Can you work these out from the model? Positions are in its coordinate system, mm. Give positions to 0.01 mm unless a question says otherwise; leave off trailing zeros. Write each loop counter-clockwise with the first axis right and the second up, starting at its lowest first coordinate (ties: lowest second). Pieces come first, ordered by that corner, then holes.
1. Suppose I cut it at C-C (x = 6). Please give me the cut outline in (y, z), and give its area (3 significant figures).
2. I'm going to push flat-ended pins straight in: pin 1 (13 mm diameter, centred on x = -29, z = 32, fed in from +Y); pin 2 (2 mm diameter, centred on x = -17, y = 4.5, fed in from -Z). Where does each tip first touch, or does it pass through?
3. Suppose I cut it at A-A (z = 16). Please give me the cut outline in (x, y), and give its area (3 significant figures).
4. If I drill on probe 1 along Z at (x, y) = (-21, 0.95); probe 2 along X at (y, z) = (0.85, 16); probe 3 along Z at (x, y) = (-13, 0.5), over which ranges is the centre line in solid material (lowest first)?
5. Thinking about a two-plate mould opening in Y: for faces 1 (the flat face through (1, 6.16, 0)), 2 (the cylindrical face through (2.479, 1.014, 28.034)), 3 (the cylindrical face through (45, 5, 0)), which applies, pulls with the +Y half, pulls with the -Y half, needs draft (parallel to the pull), parting line crosses it, or undercut?
6. Suppose I cut it at D-D (z = 37.5). Please give me the cut outline in (x, y), and give its area (3 significant figures).
7. Suppose I cut it at B-B (x = -29). Please give me the cut outline in (y, z).
```python
from build123d import *

# Parameters (mm, degrees)
SKETCH1_W               = 100
SKETCH1_H               = 100
BOSS_EXTRUDE1_DEPTH     = 2
BOSS_EXTRUDE2_DEPTH     = 100
FILLET1_R               = 10
SKETCH3_R               = 4
CUT_EXTRUDE1_DEPTH      = 3
LPATTERN1_COUNT         = 5
LPATTERN1_PITCH         = 16
LPATTERN1_COUNT_DIR2    = 2
LPATTERN1_PITCH_DIR2    = 16
MIRROR1_COPY_1_SKETCH_R = 4
MIRROR1_COPY_1_DEPTH    = 3
MIRROR1_COPY_2_SKETCH_R = 4
MIRROR1_COPY_2_DEPTH    = 3
MIRROR1_COPY_3_SKETCH_R = 4
MIRROR1_COPY_3_DEPTH    = 3
MIRROR1_COPY_4_SKETCH_R = 4
MIRROR1_COPY_4_DEPTH    = 3
MIRROR1_COPY_5_SKETCH_R = 4
MIRROR1_COPY_5_DEPTH    = 3
MIRROR1_COPY_6_SKETCH_R = 4
MIRROR1_COPY_6_DEPTH    = 3
MIRROR1_COPY_7_SKETCH_R = 4
MIRROR1_COPY_7_DEPTH    = 3
MIRROR1_COPY_8_SKETCH_R = 4
MIRROR1_COPY_8_DEPTH    = 3
MIRROR1_COPY_9_SKETCH_R = 4
MIRROR1_COPY_9_DEPTH    = 3
SKETCH4_W               = 41.2
SKETCH4_H               = 2
CUT_EXTRUDE2_DEPTH      = 101
SKETCH5_R               = 1
CUT_EXTRUDE3_DEPTH      = 59.8
LPATTERN2_COUNT         = 8
LPATTERN2_PITCH         = 13


with BuildPart() as part:
    # Sketch1 → Boss-Extrude1 (new body)
    with BuildSketch(Plane(origin=(0, 0, 0), x_dir=(1, 0, 0), z_dir=(0, 1, 0))):
        Rectangle(SKETCH1_W, SKETCH1_H)
    extrude(amount=BOSS_EXTRUDE1_DEPTH)

    # Sketch2 → Boss-Extrude2 (add)
    with BuildSketch(Plane(origin=(50, 0, 0), x_dir=(0, 0, -1), z_dir=(1, 0, 0))):
        Polygon((-3.8, 2), (-6.20177712, 6.16), (6.20177712, 6.16), (3.8, 2), align=None)
    extrude(amount=-BOSS_EXTRUDE2_DEPTH)

    # Fillet1
    fillet1_edges = [part.edges().sort_by_distance(p)[0] for p in [
        (50, 1, -50),
        (50, 1, 50),
    ]]
    fillet(fillet1_edges, radius=FILLET1_R)

    # Sketch3 → Cut-Extrude1 (cut, through all)
    with BuildSketch(Plane(origin=(0, 2, 0), x_dir=(1, 0, 0), z_dir=(0, 1, 0))):
        with Locations((35, -16)):
            Circle(SKETCH3_R)
        with Locations((27, -24)):
            Circle(SKETCH3_R)
    cut_extrude1 = extrude(amount=-CUT_EXTRUDE1_DEPTH, mode=Mode.SUBTRACT)

    # LPattern1: Cut-Extrude1 5 × 2
    with Locations(*[(-i * LPATTERN1_PITCH, 0, j * LPATTERN1_PITCH_DIR2) for i in range(LPATTERN1_COUNT) for j in range(LPATTERN1_COUNT_DIR2) if (i, j) != (0, 0)]):
        add(cut_extrude1, mode=Mode.SUBTRACT)

    # Mirror1: Cut-Extrude1 across plane
    add(cut_extrude1.mirror(Plane.XY), mode=Mode.SUBTRACT)

    # Mirror1 copy 1 sketch → Mirror1 copy 1 (cut, through all)
    with BuildSketch(Plane(origin=(0, 2, -16), x_dir=(1, 0, 0), z_dir=(0, 1, 0))):
        with Locations((35, 16)):
            Circle(MIRROR1_COPY_1_SKETCH_R)
        with Locations((27, 24)):
            Circle(MIRROR1_COPY_1_SKETCH_R)
    extrude(amount=-MIRROR1_COPY_1_DEPTH, mode=Mode.SUBTRACT)

    # Mirror1 copy 2 sketch → Mirror1 copy 2 (cut, through all)
    with BuildSketch(Plane(origin=(-16, 2, 0), x_dir=(1, 0, 0), z_dir=(0, 1, 0))):
        with Locations((35, 16)):
            Circle(MIRROR1_COPY_2_SKETCH_R)
        with Locations((27, 24)):
            Circle(MIRROR1_COPY_2_SKETCH_R)
    extrude(amount=-MIRROR1_COPY_2_DEPTH, mode=Mode.SUBTRACT)

    # Mirror1 copy 3 sketch → Mirror1 copy 3 (cut, through all)
    with BuildSketch(Plane(origin=(-16, 2, -16), x_dir=(1, 0, 0), z_dir=(0, 1, 0))):
        with Locations((35, 16)):
            Circle(MIRROR1_COPY_3_SKETCH_R)
        with Locations((27, 24)):
            Circle(MIRROR1_COPY_3_SKETCH_R)
    extrude(amount=-MIRROR1_COPY_3_DEPTH, mode=Mode.SUBTRACT)

    # Mirror1 copy 4 sketch → Mirror1 copy 4 (cut, through all)
    with BuildSketch(Plane(origin=(-32, 2, 0), x_dir=(1, 0, 0), z_dir=(0, 1, 0))):
        with Locations((35, 16)):
            Circle(MIRROR1_COPY_4_SKETCH_R)
        with Locations((27, 24)):
            Circle(MIRROR1_COPY_4_SKETCH_R)
    extrude(amount=-MIRROR1_COPY_4_DEPTH, mode=Mode.SUBTRACT)

    # Mirror1 copy 5 sketch → Mirror1 copy 5 (cut, through all)
    with BuildSketch(Plane(origin=(-32, 2, -16), x_dir=(1, 0, 0), z_dir=(0, 1, 0))):
        with Locations((35, 16)):
            Circle(MIRROR1_COPY_5_SKETCH_R)
        with Locations((27, 24)):
            Circle(MIRROR1_COPY_5_SKETCH_R)
    extrude(amount=-MIRROR1_COPY_5_DEPTH, mode=Mode.SUBTRACT)

    # Mirror1 copy 6 sketch → Mirror1 copy 6 (cut, through all)
    with BuildSketch(Plane(origin=(-48, 2, 0), x_dir=(1, 0, 0), z_dir=(0, 1, 0))):
        with Locations((35, 16)):
            Circle(MIRROR1_COPY_6_SKETCH_R)
        with Locations((27, 24)):
            Circle(MIRROR1_COPY_6_SKETCH_R)
    extrude(amount=-MIRROR1_COPY_6_DEPTH, mode=Mode.SUBTRACT)

    # Mirror1 copy 7 sketch → Mirror1 copy 7 (cut, through all)
    with BuildSketch(Plane(origin=(-48, 2, -16), x_dir=(1, 0, 0), z_dir=(0, 1, 0))):
        with Locations((35, 16)):
            Circle(MIRROR1_COPY_7_SKETCH_R)
        with Locations((27, 24)):
            Circle(MIRROR1_COPY_7_SKETCH_R)
    extrude(amount=-MIRROR1_COPY_7_DEPTH, mode=Mode.SUBTRACT)

    # Mirror1 copy 8 sketch → Mirror1 copy 8 (cut, through all)
    with BuildSketch(Plane(origin=(-64, 2, 0), x_dir=(1, 0, 0), z_dir=(0, 1, 0))):
        with Locations((35, 16)):
            Circle(MIRROR1_COPY_8_SKETCH_R)
        with Locations((27, 24)):
            Circle(MIRROR1_COPY_8_SKETCH_R)
    extrude(amount=-MIRROR1_COPY_8_DEPTH, mode=Mode.SUBTRACT)

    # Mirror1 copy 9 sketch → Mirror1 copy 9 (cut, through all)
    with BuildSketch(Plane(origin=(-64, 2, -16), x_dir=(1, 0, 0), z_dir=(0, 1, 0))):
        with Locations((35, 16)):
            Circle(MIRROR1_COPY_9_SKETCH_R)
        with Locations((27, 24)):
            Circle(MIRROR1_COPY_9_SKETCH_R)
    extrude(amount=-MIRROR1_COPY_9_DEPTH, mode=Mode.SUBTRACT)

    # Sketch4 → Cut-Extrude2 (cut, through all)
    with BuildSketch(Plane.ZY.offset(50)):
        with Locations((-29.4, 1)):
            Rectangle(SKETCH4_W, SKETCH4_H)
    extrude(amount=-CUT_EXTRUDE2_DEPTH, mode=Mode.SUBTRACT)

    # Sketch5 → Cut-Extrude3 (cut, through all)
    with BuildSketch(Plane.XY.offset(50)):
        with Locations((-46, 4)):
            Circle(SKETCH5_R)
    cut_extrude3 = extrude(amount=-CUT_EXTRUDE3_DEPTH, mode=Mode.SUBTRACT)

    # LPattern2: Cut-Extrude3 ×8
    with Locations(*[(i * LPATTERN2_PITCH, 0, 0) for i in range(1, LPATTERN2_COUNT)]):
        add(cut_extrude3, mode=Mode.SUBTRACT)


solid = part.part
```
Checks:
1. outline: (0, -8.8) - (2, -8.8) - (2, -3.8) - (3, -4.38) - (3, 4.38) - (2, 3.8) - (2, 13.35) - (0, 13.35) - close; (0, 18.65) - (2, 18.65) - (2, 29.35) - (0, 29.35) - close; (0, 34.65) - (2, 34.65) - (2, 50) - (0, 50) - close; (5, -5.53) - (6.16, -6.2) - (6.16, 6.2) - (5, 5.53) - close
1. area: 118 mm2
2. pin 1: stops at y = 2
2. pin 2: stops at z = -5.82
3. outline: (-50, 0) - (-33, 0) - (-33, 2) - (-50, 2) - close; (-25, 0) - (-17, 0) - (-17, 2) - (-25, 2) - close; (-9, 0) - (-1, 0) - (-1, 2) - (-9, 2) - close; (7, 0) - (15, 0) - (15, 2) - (7, 2) - close; (23, 0) - (31, 0) - (31, 2) - (23, 2) - close; (39, 0) - (50, 0) - (50, 2) - (39, 2) - close
3. area: 120 mm2
4. probe 1: z = -8.8 to 20, 28 to 36, 44 to 50
4. probe 2: x = -50 to -33, -25 to -17, -9 to -1, 7 to 15, 23 to 31, 39 to 50
4. probe 3: z = -8.8 to 12, 20 to 28, 36 to 50
5. face 1: pulls with the +Y half
5. face 2: needs draft
5. face 3: undercut
6. outline: (-50, 0) - (-40.12, 0) - (-40.12, 2) - (-50, 2) - close; (-33.88, 0) - (-24.12, 0) - (-24.12, 2) - (-33.88, 2) - close; (-17.88, 0) - (-8.12, 0) - (-8.12, 2) - (-17.88, 2) - close; (-1.88, 0) - (7.88, 0) - (7.88, 2) - (-1.88, 2) - close; (14.12, 0) - (23.88, 0) - (23.88, 2) - (14.12, 2) - close; (30.12, 0) - (50, 0) - (50, 2) - (30.12, 2) - close
6. area: 138 mm2
7. outline: (0, -8.8) - (2, -8.8) - (2, -3.8) - (6.16, -6.2) - (6.16, 6.2) - (2, 3.8) - (2, 12) - (0, 12) - close; (0, 20) - (2, 20) - (2, 28) - (0, 28) - close; (0, 36) - (2, 36) - (2, 50) - (0, 50) - close
